Part model, mm, in its own coordinate system. Coordinates: 2 decimals unless noted, no trailing zeros. Order: outer loops, then holes, each group sorted by start corner. A loop starts at its lowest first (then second) coordinate and runs counter-clockwise, first axis right, second up.
from build123d import *

# Parameters (mm, degrees)
CORTE_EXTRUS_O4_START  = -1
ESBO_O2_R              = 1.5
CORTE_EXTRUS_O4_DEPTH  = 7
CORTE_EXTRUS_O9_START  = -4
CORTE_EXTRUS_O9_DEPTH  = 7
PADR_OCIRCULAR1_COUNT  = 4
ESBO_O7_R              = 4
CORTE_EXTRUS_O10_DEPTH = 10


with BuildPart() as part:
    # Esboço1 → Revolução1 (revolve)
    with BuildSketch(Plane.XY):
        with BuildLine():
            Line((1.1, 5), (1.1, 0))
            Line((1.1, 0), (38, 0))
            Line((38, 0), (38, 3))
            Line((38, 3), (5.9, 3))
            ThreePointArc((5.9, 3), (4.556497116, 3.556497116), (4, 4.9))
            Line((4, 4.9), (4, 5))
            Line((4, 5), (1.1, 5))
        make_face()
    revolve(axis=Axis((0, 0, 0), (0, 1, 0)))

    # Esboço2 → Corte-extrusão4 (cut)
    with BuildSketch(Plane(origin=(0, 0, 0), x_dir=(1, 0, 0), z_dir=(0, 1, 0)).offset(CORTE_EXTRUS_O4_START)):
        with Locations((0, 20)):
            Circle(ESBO_O2_R)
    corte_extrus_o4 = extrude(amount=CORTE_EXTRUS_O4_DEPTH, mode=Mode.SUBTRACT)

    # Esboço6 → Corte-extrusão9 (cut)
    with BuildSketch(Plane(origin=(0, 3, 0), x_dir=(1, 0, 0), z_dir=(0, 1, 0)).offset(CORTE_EXTRUS_O9_START)):
        with BuildLine():
            Line((3, 27.838821814), (3, 5.080354318))
            ThreePointArc((3, 5.080354318), (4.171930009, 4.171930009), (5.080354318, 3))
            Line((5.080354318, 3), (27.838821814, 3))
            ThreePointArc((27.838821814, 3), (19.798989873, 19.798989873), (3, 27.838821814))
        make_face()
    corte_extrus_o9 = extrude(amount=CORTE_EXTRUS_O9_DEPTH, mode=Mode.SUBTRACT)

    # PadrãoCircular1: Corte-extrusão4, Corte-extrusão9 ×4 about axis
    padr_ocircular1_axis = Axis((0, 0, 0), (0, 1, 0))
    for i in range(1, PADR_OCIRCULAR1_COUNT):
        add(corte_extrus_o4.rotate(padr_ocircular1_axis, i * 360 / PADR_OCIRCULAR1_COUNT), mode=Mode.SUBTRACT)
        add(corte_extrus_o9.rotate(padr_ocircular1_axis, i * 360 / PADR_OCIRCULAR1_COUNT), mode=Mode.SUBTRACT)

    # Esboço7 → Corte-extrusão10 (cut)
    with BuildSketch(Plane(origin=(0, 3, 0), x_dir=(1, 0, 0), z_dir=(0, 1, 0))):
        with Locations((0, 33)):
            Circle(ESBO_O7_R)
    extrude(amount=-CORTE_EXTRUS_O10_DEPTH, mode=Mode.SUBTRACT)


solid = part.part
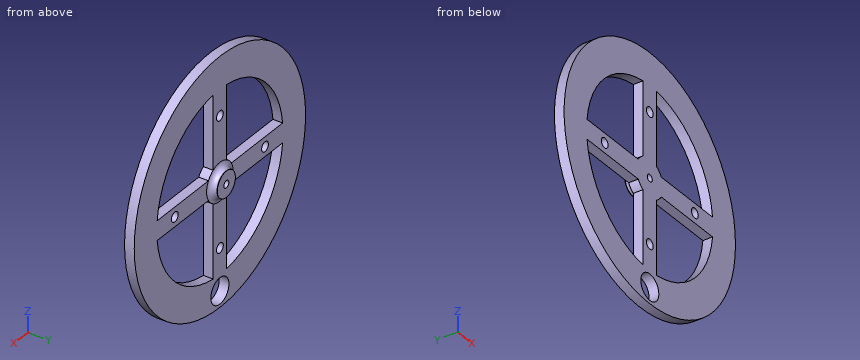
Q1. Wall check: line 1 along Z through (x, y) = (0, 1.3); line 2 along X through (y, z) = (2.75, 0); line 3 along Z through (x, y) = (-12.5, 2.4). Give the ranges that are in metal, low to high.
Results list:
line 1: z = -38 to -37, -29 to -21.5, -18.5 to -1.1, 1.1 to 18.5, 21.5 to 38
line 2: x = -38 to -21.5, -18.5 to -1.1, 1.1 to 18.5, 21.5 to 38
line 3: z = -35.89 to -25.05, -3 to 3, 25.05 to 35.89
Q2. Cut at D-D on x = 25. Write the cut outline in (y, z), and give its area (3 significant figures).
Results list:
outline: (0, -28.62) - (3, -28.62) - (3, -12.61) - (0, -12.61) - close; (0, -3) - (3, -3) - (3, 3) - (0, 3) - close; (0, 12.61) - (3, 12.61) - (3, 28.62) - (0, 28.62) - close
area: 114 mm2
Q3. Cut at A-A on z = 0. Write the cut outline in (x, y).
Results list:
outline: (-38, 0) - (-21.5, 0) - (-21.5, 3) - (-38, 3) - close; (-18.5, 0) - (-1.1, 0) - (-1.1, 5) - (-4, 5) - (-4, 4.9) arc R1.9 cw to (-5.9, 3) - (-18.5, 3) - close; (1.1, 0) - (18.5, 0) - (18.5, 3) - (5.9, 3) arc R1.9 cw to (4, 4.9) - (4, 5) - (1.1, 5) - close; (21.5, 0) - (38, 0) - (38, 3) - (21.5, 3) - close
Q4. Cut at B-B on x = 0. Write the cut outline in (y, z), and give its area (3 significant figures).
Results list:
outline: (0, -38) - (3, -38) - (3, -37) - (0, -37) - close; (0, -29) - (3, -29) - (3, -21.5) - (0, -21.5) - close; (0, -18.5) - (3, -18.5) - (3, -5.9) arc R1.9 cw to (4.9, -4) - (5, -4) - (5, -1.1) - (0, -1.1) - close; (0, 1.1) - (5, 1.1) - (5, 4) - (4.9, 4) arc R1.9 cw to (3, 5.9) - (3, 18.5) - (0, 18.5) - close; (0, 21.5) - (3, 21.5) - (3, 38) - (0, 38) - close
area: 193 mm2
Q5. Cut at C-C on z = -17. Write the cut outline in (x, y).
Results list:
outline: (-33.99, 0) - (-22.25, 0) - (-22.25, 3) - (-33.99, 3) - close; (-3, 0) - (3, 0) - (3, 3) - (-3, 3) - close; (22.25, 0) - (33.99, 0) - (33.99, 3) - (22.25, 3) - close
Q6. Pin check, flat tips, straight feed: pin 1 Ø1.5 at (x, y) = (-17.5, 1.5) entering from +Z; pin 2 Ø2 at (y, z) = (2, 26.5) entering from +X; pin 3 Ø2.5 at (x, y) = (-15, 1) entering from -Z; pin 4 Ø3.5 at (x, z) = (-20, 0) entering from -Y. Stop position of each tip, or through.
Results list:
pin 1: stops at z = 34.11
pin 2: stops at x = 28.17
pin 3: stops at z = -35.43
pin 4: stops at y = 0
